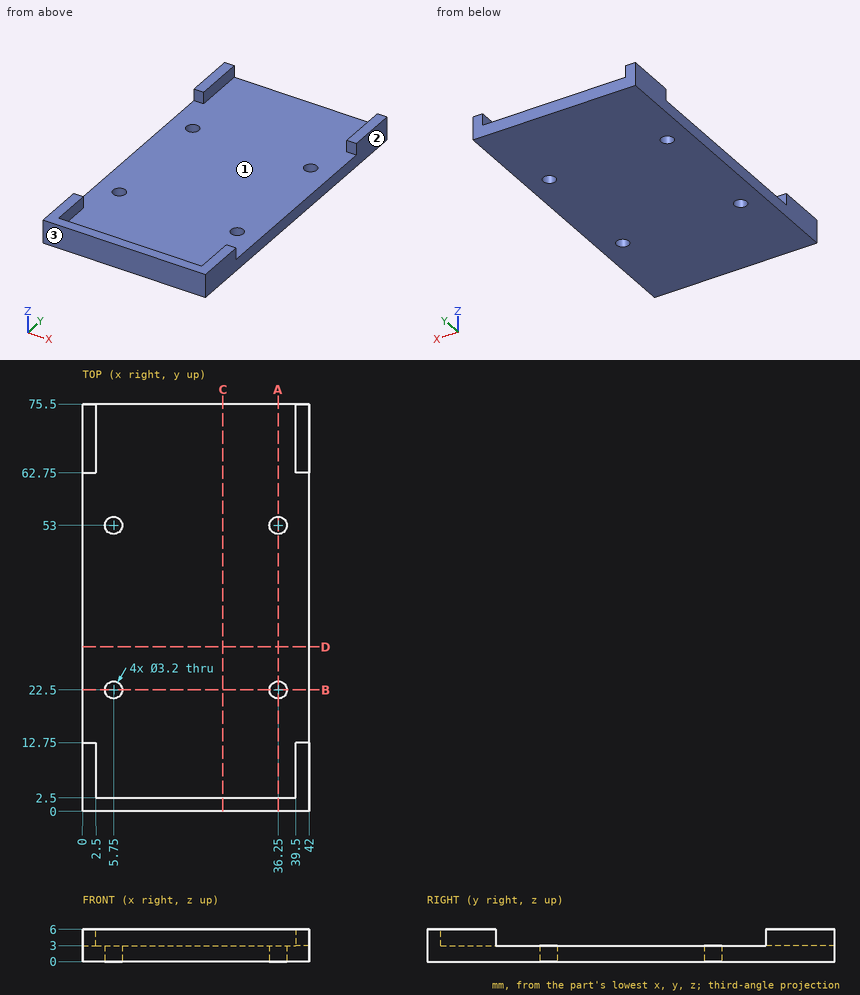
Check sheet for the drawn part. Datum: minimum x, y, z corner. Units: mm. Coordinates: 2 decimals unless noted, no trailing zeros. Loops run counter-clockwise (first coordinate to the right, second up) from the corner with the lowest first, then second, coordinate; pieces in that order, holes last. Notation, with made-up numbers: (70.25, 16) - (99.25, 16) arc R28 ccw to (99.25, 43) - close; hole circle Ø6 at (56.25, 43). An arc over 180 degrees is marked (long way). Put each result on its own line as item: value.
Item 1: Section check B-B (y = 22.5). Enter the section's corners in (x, z), then the cut area to 3 significant figures.
Conclusion:
outline: (0, 0) - (4.15, 0) - (4.15, 3) - (0, 3) - close; (7.35, 0) - (34.65, 0) - (34.65, 3) - (7.35, 3) - close; (37.85, 0) - (42, 0) - (42, 3) - (37.85, 3) - close
area: 107 mm2
Item 2: Section check A-A (x = 36.25). Enter the section's corners in (y, z), then the cut area to 3 significant figures.
Conclusion:
outline: (0, 0) - (20.9, 0) - (20.9, 3) - (2.5, 3) - (2.5, 6) - (0, 6) - close; (24.1, 0) - (51.4, 0) - (51.4, 3) - (24.1, 3) - close; (54.6, 0) - (75.5, 0) - (75.5, 3) - (54.6, 3) - close
area: 215 mm2
Item 3: Draft check along X on the marked faces 1, 2 and 3. Enter one of: pulls with the +X half, pulls with the -X half, needs draft (parallel to the pull), parting line crosses it, or undercut.
Conclusion:
face 1: undercut
face 2: pulls with the +X half
face 3: needs draft
Item 4: Section check C-C (x = 26). Enter the section's corners in (y, z), then the cut area to 3 significant figures.
Conclusion:
outline: (0, 0) - (75.5, 0) - (75.5, 3) - (2.5, 3) - (2.5, 6) - (0, 6) - close
area: 234 mm2
Item 5: Section check D-D (y = 30.5). Enter the section's corners in (x, z).
Conclusion:
outline: (0, 0) - (42, 0) - (42, 3) - (0, 3) - close
Item 6: Scan lines: line 1 along Y through (x, z) = (5.75, 1.4); line 2 along X through (y, z) = (9, 3.85); line 3 along Z through (x, y) = (24.5, 13.5). Record each from-to range of solid material in increasing order.
Conclusion:
line 1: y = 0 to 20.9, 24.1 to 51.4, 54.6 to 75.5
line 2: x = 0 to 2.5, 39.5 to 42
line 3: z = 0 to 3
Item 7: Gauge pin test, flat end, axial feed: pin 1 Ø1.5 at (x, y) = (12.5, 10.5) entering from +Z. Record the tip position at first contact, or that the pin passes through.
Conclusion:
pin 1: stops at z = 3
